Source: CAD feature listing. Evaluate the final solid. Frame: model axes, mm. Coordinates: 2 decimals unless noted, no trailing zeros. Write each loop counter-clockwise with the first axis right and the second up, starting at its lowest first coordinate (ties: lowest second). Pieces come first, ordered by that corner, then holes. Notation, with made-up numbers: (57, 89.5) - (95, 89.5) arc R37 cw to (95, 128.5) - close; hole circle Ø3 at (-3.5, -36). An arc over 180 degrees is marked (long way). One line per item, written item: value.
from build123d import *

# Parameters (mm, degrees)
SKETCH_1_R      = 3.35
EXTRUDE_1_DEPTH = 2.2
CHAMFER_1_SIZE  = 0.4


with BuildPart() as part:
    # 草图1 → 凸台-拉伸1 (new body)
    with BuildSketch(Plane.XY):
        Polygon((5.035878056, -2.703688629), (4.859402065, 3.009354013), (-0.176475992, 5.713042642), (-5.035878056, 2.703688629), (-4.859402065, -3.009354013), (0.176475992, -5.713042642), align=None)
        Circle(SKETCH_1_R, mode=Mode.SUBTRACT)
    extrude(amount=EXTRUDE_1_DEPTH)

    # 倒角1
    chamfer_1_edges = [part.edges().sort_by_distance(p)[0] for p in [
        (2.341463036, 4.361198327, 2.2),
        (-2.606177024, 4.208365635, 2.2),
        (-4.94764006, -0.152832692, 2.2),
        (-2.341463036, -4.361198327, 2.2),
        (2.606177024, -4.208365635, 2.2),
        (-2.341463036, -4.361198327, 0),
        (-4.94764006, -0.152832692, 0),
        (-2.606177024, 4.208365635, 0),
        (4.94764006, 0.152832692, 2.2),
        (2.341463036, 4.361198327, 0),
        (2.606177024, -4.208365635, 0),
    ]]
    chamfer(chamfer_1_edges, length=CHAMFER_1_SIZE)


solid = part.part
1) Section query D-D on x = 1.5. Output: boundary loops of the cut face in (y, z), then the cut area to 3 significant figures.
Values found:
outline: (-4.89, 0.4) - (-4.42, 0) - (-3, 0) - (-3, 2.2) - (-4.42, 2.2) - (-4.89, 1.8) - close; (3, 0) - (4.36, 0) - (4.81, 0.4) - (4.81, 1.8) - (4.36, 2.2) - (3, 2.2) - close
area: 7.80 mm2
2) Material intervals for line 1 (X direction, y = 2.5, z = 1.1); line 2 (Y direction, x = 0, z = 1.3); line 3 (Y direction, x = 0.5, z = 0.95), sorted ascending.
Values found:
line 1: -5.03 to -2.23, 2.23 to 4.88
line 2: -5.62 to -3.35, 3.35 to 5.62
line 3: -5.51 to -3.31, 3.31 to 5.35
3) Section query C-C on x = -3. Output: boundary loops of the cut face in (y, z).
Values found:
outline: (-4.01, 0.4) - (-3.55, 0) - (-1.49, 0) - (-1.49, 2.2) - (-3.55, 2.2) - (-4.01, 1.8) - close; (1.49, 0) - (3.49, 0) - (3.96, 0.4) - (3.96, 1.8) - (3.49, 2.2) - (1.49, 2.2) - close
4) Section query A-A on y = 1. Output: boundary loops of the cut face in (x, z).
Values found:
outline: (-4.98, 0.4) - (-4.58, 0) - (-3.2, 0) - (-3.2, 2.2) - (-4.58, 2.2) - (-4.98, 1.8) - close; (3.2, 0) - (4.92, 0) - (4.92, 1.8) - (4.52, 2.2) - (3.2, 2.2) - close
5) Draft query along X for faces 1 (the flat face through (3.35, -1.09, 0)), 2 (the cylindrical face through (-3.347, 0.147, 1.085)), 3 (the flat face through (2.57, -4.23, 1.09)), 4 (the flat face through (-2.47, 4.06, 2)). Return one class per face: released by +X, released by -X, zero draft, split by the parting line, or undercut.
Values found:
face 1: zero draft
face 2: undercut
face 3: released by +X
face 4: released by -X
6) Section query B-B on z = 1.15. Output: boundary loops of the cut face in (x, y), then the cut area to 3 significant figures.
Values found:
outline: (-5.04, 2.7) - (-4.86, -3.01) - (0.18, -5.71) - (5.04, -2.7) - (4.86, 3.01) - (-0.18, 5.71) - close; hole circle Ø6.7 at (0, 0)
area: 49.6 mm2
